Read the model definition and answer for the solid it produces. Units are mm, in the model's axes. A direction names the side the tool comes from. Coordinates: 2 decimals unless noted, no trailing zeros. Order: outer loops, then holes, each group sorted by start corner. A loop starts at its lowest first (then second) coordinate and runs counter-clockwise, first axis right, second up.
from build123d import *
from build123d.topology import SkipClean

# Parameters (mm, degrees)
MAIN_DEPTH            = 2.5
ESQUISSE2_R           = 2.5
ORIGINALBRACKET_DEPTH = 2
ESQUISSE3_R           = 1.3
FIXINGHOLE_DEPTH      = 37.183559803


with BuildPart() as part:
    # Esquisse1 → Main (new body)
    with BuildSketch(Plane.XY):
        with BuildLine():
            Line((0.8, 7.959899497), (30.5, 4.974937186))
            ThreePointArc((30.5, 4.974937186), (35, 0), (30.5, -4.974937186))
            Line((30.5, -4.974937186), (0.8, -7.959899497))
            ThreePointArc((0.8, -7.959899497), (-8, 0), (0.8, 7.959899497))
        make_face()
        with BuildLine():
            Line((0.336544343, 3.534011588), (16.539602446, 1.990992444))
            ThreePointArc((16.539602446, 1.990992444), (18.35, 0), (16.539602446, -1.990992444))
            Line((16.539602446, -1.990992444), (0.336544343, -3.534011588))
            ThreePointArc((0.336544343, -3.534011588), (-3.55, 0), (0.336544343, 3.534011588))
        make_face(mode=Mode.SUBTRACT)
    extrude(amount=MAIN_DEPTH)

    # Esquisse2 → OriginalBracket (add)
    with SkipClean():  # the faces are left unmerged after this step: merging them gives an invalid solid
        with BuildSketch(Plane(origin=(0, 0, 0), x_dir=(-1, 0, 0), z_dir=(0, 0, -1))):
            with BuildLine():
                Line((-0.8, -7.959899497), (-30.5, -4.974937186))
                ThreePointArc((-30.5, -4.974937186), (-35, 0), (-30.5, 4.974937186))
                Line((-30.5, 4.974937186), (-0.8, 7.959899497))
                ThreePointArc((-0.8, 7.959899497), (8, 0), (-0.8, -7.959899497))
            make_face()
            Circle(ESQUISSE2_R, mode=Mode.SUBTRACT)
        extrude(amount=ORIGINALBRACKET_DEPTH)

    # Esquisse3 → FixingHole (cut, through all)
    with SkipClean():  # the faces are left unmerged after this step: merging them gives an invalid solid
        with BuildSketch(Plane.XY.offset(2.5)):
            with Locations((30, 0)):
                Circle(ESQUISSE3_R)
            with Locations((25, 0)):
                Circle(ESQUISSE3_R)
        extrude(amount=-FIXINGHOLE_DEPTH, mode=Mode.SUBTRACT)


solid = part.part
Q1. Which of the six approach directions +Z, -Z, +X, -X, +Y, -Y give full straight-line access (tool end or side, diameter ignored) to faces 1 (the flat face through (7, 0, 0)), 2 (the cylindrical face through (23.7, 0.06, 0.28))?
Q2. The part is cut by section C-C, the plane z = 1.15. Determine the outline of the cut face in (x, y), then the cut area to 3 significant figures.
Q3. The part is cut by section A-A, the plane y = 0. Determine the outline of the cut face in (x, z).
Q4. The part is cut by section D-D, the plane x = 5. Determine the outline of the cut face in (y, z), then the cut area to 3 significant figures.
Q5. Straight lines are drawn through the part: L1, parallel to Y at x = 0, z = -0.7; L2, parallel to X at y = -1, z = -0.75; L3, parallel to Y at x = 0, z = 1.85. For each, find the intervals that lie inside material, in ascending order.
Q6. The part is cut by section B-B, the plane x = 25. Determine the outline of the cut face in (y, z), then the cut area to 3 significant figures.
Q7. Each of these flat-tipped pins is pushed along its axis until it touches: P1, Ø4.5, axis at x = 0, y = 0, coming from the +Z side; P2, Ø2, axis at x = 4.5, y = -0.5, coming from the +Z side; P3, Ø2, axis at x = 3, z = 1, coming from the +Y side. Where does it stop, or does it pass through?
Q8. Determine the mould class of faces 3 (the cylindrical face through (0.54, -2.44, -0.99)), 4 (the flat face through (13, 0, -2)) for opening direction X: +X half, -X half, draft (parallel to the pull), parting line (faces both ways), or undercut.
Computed values:
1. face 1: +Z
1. face 2: +Z, -Z
2. outline: (0.8, -7.96) - (30.5, -4.97) arc R5 ccw to (30.5, 4.97) - (0.8, 7.96) arc R8 ccw (long way) to start; hole (0.34, -3.53) - (16.54, -1.99) arc R2 ccw to (16.54, 1.99) - (0.34, 3.53) arc R3.55 ccw (long way) to start; hole circle Ø2.6 at (25, 0); hole circle Ø2.6 at (30, 0)
2. area: 404 mm2
3. outline: (-8, -2) - (-2.5, -2) - (-2.5, 0) - (-3.55, 0) - (-3.55, 2.5) - (-8, 2.5) - close; (2.5, -2) - (23.7, -2) - (23.7, 2.5) - (18.35, 2.5) - (18.35, 0) - (2.5, 0) - close; (26.3, -2) - (28.7, -2) - (28.7, 2.5) - (26.3, 2.5) - close; (31.3, -2) - (35, -2) - (35, 2.5) - (31.3, 2.5) - close
4. outline: (-7.54, -2) - (7.54, -2) - (7.54, 2.5) - (3.09, 2.5) - (3.09, 0) - (-3.09, 0) - (-3.09, 2.5) - (-7.54, 2.5) - close
4. area: 52.4 mm2
5. L1: y = -8 to -2.5, 2.5 to 8
5. L2: x = -7.94 to -2.29, 2.29 to 24.17, 25.83 to 29.17, 30.83 to 34.9
5. L3: y = -8 to -3.55, 3.55 to 8
6. outline: (-5.53, -2) - (-1.3, -2) - (-1.3, 2.5) - (-5.53, 2.5) - close; (1.3, -2) - (5.53, -2) - (5.53, 2.5) - (1.3, 2.5) - close
6. area: 38.0 mm2
7. P1: passes through
7. P2: stops at z = 0
7. P3: stops at y = 7.84
8. face 3: undercut
8. face 4: draft
